```python
from build123d import *

# Parameters (mm, degrees)
SKETCH2_R                = 304.8
BOSS_EXTRUDE1_DEPTH      = 3.175
BOSS_EXTRUDE1_DEPTH_BACK = 3.175
SKETCH5_R                = 317.5
SKETCH5_R_2              = 304.8
BOSS_EXTRUDE2_DEPTH      = 50.8
BOSS_EXTRUDE2_DEPTH_BACK = 50.8
SKETCH6_R                = 4.7625
CUT_EXTRUDE1_DEPTH       = 54.975


with BuildPart() as part:
    # Sketch2 → Boss-Extrude1 (new body, two sides)
    with BuildSketch(Plane.XY) as boss_extrude1_sk:
        Circle(SKETCH2_R)
        with BuildLine():
            Line((25.4, -252.726809025), (25.4, -71.842048969))
            ThreePointArc((25.4, -71.842048969), (38.1, -65.991135768), (49.517039467, -57.91806974))
            Line((49.517039467, -57.91806974), (206.167836833, -148.360449769))
            ThreePointArc((206.167836833, -148.360449769), (127, -219.970452561), (25.4, -252.726809025))
        make_face(mode=Mode.SUBTRACT)
        with BuildLine():
            Line((231.567836833, -104.366359256), (74.917039467, -13.923979228))
            ThreePointArc((74.917039467, -13.923979228), (76.2, 0), (74.917039467, 13.923979228))
            Line((74.917039467, 13.923979228), (231.567836833, 104.366359256))
            ThreePointArc((231.567836833, 104.366359256), (254, 0), (231.567836833, -104.366359256))
        make_face(mode=Mode.SUBTRACT)
        with BuildLine():
            Line((206.167836833, 148.360449769), (49.517039467, 57.91806974))
            ThreePointArc((49.517039467, 57.91806974), (38.1, 65.991135768), (25.4, 71.842048969))
            Line((25.4, 71.842048969), (25.4, 252.726809025))
            ThreePointArc((25.4, 252.726809025), (127, 219.970452561), (206.167836833, 148.360449769))
        make_face(mode=Mode.SUBTRACT)
        with BuildLine():
            Line((-25.4, 252.726809025), (-25.4, 71.842048969))
            ThreePointArc((-25.4, 71.842048969), (-38.1, 65.991135768), (-49.517039467, 57.91806974))
            Line((-49.517039467, 57.91806974), (-206.167836833, 148.360449769))
            ThreePointArc((-206.167836833, 148.360449769), (-127, 219.970452561), (-25.4, 252.726809025))
        make_face(mode=Mode.SUBTRACT)
        with BuildLine():
            Line((-231.567836833, 104.366359256), (-74.917039467, 13.923979228))
            ThreePointArc((-74.917039467, 13.923979228), (-76.2, 0), (-74.917039467, -13.923979228))
            Line((-74.917039467, -13.923979228), (-231.567836833, -104.366359256))
            ThreePointArc((-231.567836833, -104.366359256), (-254, 0), (-231.567836833, 104.366359256))
        make_face(mode=Mode.SUBTRACT)
        with BuildLine():
            Line((-206.167836833, -148.360449769), (-49.517039467, -57.91806974))
            ThreePointArc((-49.517039467, -57.91806974), (-38.1, -65.991135768), (-25.4, -71.842048969))
            Line((-25.4, -71.842048969), (-25.4, -252.726809025))
            ThreePointArc((-25.4, -252.726809025), (-127, -219.970452561), (-206.167836833, -148.360449769))
        make_face(mode=Mode.SUBTRACT)
    extrude(amount=BOSS_EXTRUDE1_DEPTH)
    extrude(boss_extrude1_sk.sketch, amount=-BOSS_EXTRUDE1_DEPTH_BACK)

    # Sketch5 → Boss-Extrude2 (add, two sides)
    with BuildSketch(Plane.XY) as boss_extrude2_sk:
        Circle(SKETCH5_R)
        Circle(SKETCH5_R_2, mode=Mode.SUBTRACT)
    extrude(amount=BOSS_EXTRUDE2_DEPTH)
    extrude(boss_extrude2_sk.sketch, amount=-BOSS_EXTRUDE2_DEPTH_BACK)

    # Sketch6 → Cut-Extrude1 (cut, through all)
    with BuildSketch(Plane.XY.offset(3.175)):
        with Locations((0, 50.8)):
            Circle(SKETCH6_R)
        with Locations((43.994090512, 25.4)):
            Circle(SKETCH6_R)
        with Locations((43.994090512, -25.4)):
            Circle(SKETCH6_R)
        with Locations((0, -50.8)):
            Circle(SKETCH6_R)
        with Locations((-43.994090512, -25.4)):
            Circle(SKETCH6_R)
        with Locations((-43.994090512, 25.4)):
            Circle(SKETCH6_R)
    extrude(amount=-CUT_EXTRUDE1_DEPTH, mode=Mode.SUBTRACT)


solid = part.part
```
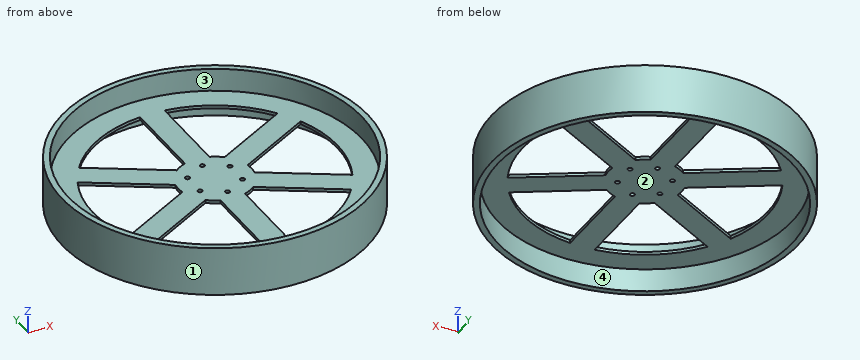
Part model, mm, in its own coordinate system. Face numbers are marked on the shaded views. A direction names the side the tool comes from. Give positions to 0.01 mm unless a question says otherwise; leave off trailing zeros. Write each loop counter-clockwise with the first axis right and the second up, starting at its lowest first coordinate (ties: lowest second). Pieces come first, ordered by that corner, then holes. Notation, with made-up numbers: (1.5, -8.75) -> (13.5, -8.75) arc R12 cw to (13.5, 12.25) -> close; hole circle Ø11 at (-6, 8). An arc over 180 degrees is marked (long way). Put each result on its own line as item: value. Start each with the question number.
Item 1: Cut at D-D (y = 264.5). List the corners of the cut face in (x, z) (3 decimals), then the cut area to 3 significant figures.
Item 2: Pin check, flat tips, straight feed: pin 1 Ø6 at (y, z) = (-88, -6.5) entering from +X; pin 2 Ø15 at (x, y) = (-43.99, 25.4) entering from +Z (3 decimals); pin 3 Ø5 at (y, z) = (174.5, -0.5) entering from +X (3 decimals); pin 4 Ø7.5 at (x, y) = (0, -50.8) entering from -Z. Stop position of each tip, or through.
Item 3: Wall check: L1, parallel to Y at x = 0, z = 17; L2, parallel to Z at x = 167, y = 230 (3 decimals); L3, parallel to Y at x = 280.5, z = 31.5. Give the ranges that are in metal, low to high. Write a range as [from, to].
Item 4: Cut at A-A (y = 0). List the corners of the cut face in (x, z) (3 decimals), then the cut area to 3 significant figures.
Item 5: Cut at B-B (x = -61). List the corners of the cut face in (y, z) (3 decimals), then the cut area to 3 significant figures.
Item 6: Which spindle directions (+Z, -Z, +X, -X, +Y, -Y) get a long thin tool onto all of the face, cutting with end or side? Do the marked faces 3 and 4. Say none if no direction does.
Item 7: Pull direction X, two halves, no side cores. Call the marked faces 1 and 2: pulls with the +X half, pulls with the -X half, needs draft (parallel to the pull), parting line crosses it, or undercut.
Item 8: Cut at C-C (z = 25). List the corners of the cut face in (x, y).
Answer list:
1. outline: (-175.63, -50.8) -> (-151.469, -50.8) -> (-151.469, -3.175) -> (151.469, -3.175) -> (151.469, -50.8) -> (175.63, -50.8) -> (175.63, 50.8) -> (151.469, 50.8) -> (151.469, 3.175) -> (-151.469, 3.175) -> (-151.469, 50.8) -> (-175.63, 50.8) -> close
1. area: 6,830 mm2
2. pin 1: stops at x = 305.91
2. pin 2: stops at z = 3.175
2. pin 3: stops at x = 266.875
2. pin 4: passes through
3. L1: y = [-317.5, -304.8], [304.8, 317.5]
3. L2: z = [-3.175, 3.175]
3. L3: y = [-148.75, -119.26], [119.26, 148.75]
4. outline: (-317.5, -50.8) -> (-304.8, -50.8) -> (-304.8, -3.175) -> (-254, -3.175) -> (-254, 3.175) -> (-304.8, 3.175) -> (-304.8, 50.8) -> (-317.5, 50.8) -> close; (-76.2, -3.175) -> (76.2, -3.175) -> (76.2, 3.175) -> (-76.2, 3.175) -> close; (254, -3.175) -> (304.8, -3.175) -> (304.8, -50.8) -> (317.5, -50.8) -> (317.5, 50.8) -> (304.8, 50.8) -> (304.8, 3.175) -> (254, 3.175) -> close
4. area: 4,190 mm2
5. outline: (-311.585, -50.8) -> (-298.634, -50.8) -> (-298.634, -3.175) -> (-246.566, -3.175) -> (-246.566, 3.175) -> (-298.634, 3.175) -> (-298.634, 50.8) -> (-311.585, 50.8) -> close; (-64.548, -3.175) -> (64.548, -3.175) -> (64.548, 3.175) -> (-64.548, 3.175) -> close; (246.566, -3.175) -> (298.634, -3.175) -> (298.634, -50.8) -> (311.585, -50.8) -> (311.585, 50.8) -> (298.634, 50.8) -> (298.634, 3.175) -> (246.566, 3.175) -> close
5. area: 4,110 mm2
6. face 3: +Z
6. face 4: -Z
7. face 1: parting line crosses it
7. face 2: undercut
8. outline: circle Ø635 at (0, 0); hole circle Ø609.6 at (0, 0)
